Read the model definition and answer for the solid it produces. Units are mm, in the model's axes. Give positions to 0.01 mm unless a question says otherwise; leave off trailing zeros. Write each loop counter-clockwise with the first axis right and the second up, starting at its lowest first coordinate (ties: lowest second). Pieces come first, ordered by that corner, then holes. Notation, with made-up numbers: (80, 38) - (104, 38) arc R20 ccw to (104, 77) - close; hole circle Ø10 at (56, 81). An arc over 180 degrees is marked (long way). Answer as CSV lines item,"result".
```python
from build123d import *

# Parameters (mm, degrees)
F1_DEPTH = 3.175
F2_R     = 1.27


# Not quite as in the source:
# - a feature names something its author has since deleted; it is built from what else it names


with BuildPart() as f1:
    # F0 (on Top) → F1 (new body)
    with BuildSketch(Plane.XY):
        with BuildLine():
            Line((0, 7.62), (0, 12.7))
            ThreePointArc((0, 12.7), (-8.9802561211, 8.9802561211), (-12.7, 0))
            Line((-12.7, 0), (-7.62, 0))
            ThreePointArc((-7.62, 0), (-5.3881536726, 5.3881536726), (0, 7.62))
        make_face()
        with BuildLine():
            ThreePointArc((-12.7, 0), (-8.9802561211, 8.9802561211), (0, 12.7))
            Line((0, 12.7), (0, 48.26))
            ThreePointArc((0, 48.26), (-34.1249732601, 34.1249732601), (-48.26, 0))
            Line((-48.26, 0), (-12.7, 0))
        make_face()
        with BuildLine():
            ThreePointArc((-48.26, 0), (-34.1249732601, 34.1249732601), (0, 48.26))
            Line((0, 48.26), (0, 53.34))
            ThreePointArc((0, 53.34), (-37.7170757085, 37.7170757085), (-53.34, 0))
            Line((-53.34, 0), (-48.26, 0))
        make_face()
    extrude(amount=F1_DEPTH)

    # F2
    f2_edges = [f1.edges().sort_by_distance(p)[0] for p in [
        (-7.62, 0, 1.5875),
        (0, 7.62, 1.5875),
    ]]
    fillet(f2_edges, radius=F2_R)


solid = f1.part
```
(1) A cutting plane is placed at B-B (x = -25). Write down the section's boundary in (y, z) (3 decimals).
Worked out:
outline,"(0, 0) - (47.119, 0) - (47.119, 3.175) - (0, 3.175) - close"
(2) A cutting plane is placed at C-C (y = 33). Write down the section's boundary in (x, z) (3 decimals).
Worked out:
outline,"(-41.907, 0) - (0, 0) - (0, 3.175) - (-41.907, 3.175) - close"
(3) A cutting plane is placed at A-A (z = 0.8). Write down the section's boundary in (x, y), and give its area (3 significant figures).
Worked out:
outline,"(-53.34, 0) - (-8.8, 0) arc R1.27 ccw to (-7.54, 1.09) arc R7.62 cw to (-1.09, 7.54) arc R1.27 ccw to (0, 8.8) - (0, 53.34) arc R53.34 ccw to start"
area,"2,190 mm^2"
(4) Each of these flat-tipped pins is pushed along its axis until it touches: P1, Ø1.5, axis at y = 12.5, z = 2, coming from the -X side; P2, Ø3, axis at x = -31.5, y = 21.5, coming from the -Z side. Where does it stop, or does it pass through?
Worked out:
P1,"stops at x = -52.03"
P2,"stops at z = 0"
(5) Find the intervals of material crossed by L1, parallel to X at y = 40, z = 2.45; L2, parallel to X at y = 43.5, z = 0.4; L3, parallel to Y at x = -30.5, z = 1, in increasing order.
Worked out:
L1,"x = -35.29 to 0"
L2,"x = -30.87 to 0"
L3,"y = 0 to 43.76"
